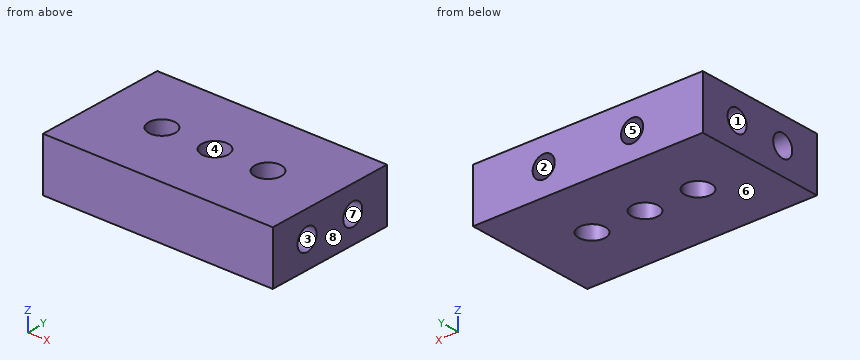
```python
from build123d import *

# Parameters (mm, degrees)
SKETCH_1_W                  = 26
SKETCH_1_H                  = 15
EXTRUDE_1_DEPTH             = 5
SKETCH_2_W                  = 26
SKETCH_2_H                  = 15
EXTRUDE_2_DEPTH             = 1
HOLE_WIZARD_M3_1_AT_2_COUNT = 2
HOLE_WIZARD_M3_1_AT_2_PITCH = 6
SKETCH_5_R                  = 1.5
CUT_EXTRUDE_1_DEPTH         = 7
HOLE_WIZARD_M3_2_D          = 2.5
HOLE_WIZARD_M3_2_DEPTH      = 7
HOLE_WIZARD_M3_2_TIP        = 0.751075774


with BuildPart() as part:
    # 草图1 → 凸台-拉伸1 (new body)
    with BuildSketch(Plane.XY):
        Rectangle(SKETCH_1_W, SKETCH_1_H)
    extrude(amount=EXTRUDE_1_DEPTH)

    # 草图2 → 凸台-拉伸2 (add)
    with BuildSketch(Plane.XY.offset(5)):
        Rectangle(SKETCH_2_W, SKETCH_2_H)
    extrude(amount=EXTRUDE_2_DEPTH)

    # 草图4 → M3 螺纹孔1 (revolve, cut)
    with BuildSketch(Plane(origin=(-13, -3, 3), x_dir=(0, 0, 1), z_dir=(0, 1, 0))):
        Polygon((0, 0), (0, 5.751075774), (1.25, 5), (1.25, 0), align=None)
    hole_wizard_m3_1 = revolve(axis=Axis((-19.35, -3, 3), (1, 0, 0)), mode=Mode.SUBTRACT)

    # M3 螺纹孔1 at 2: M3 螺纹孔1 ×2
    with Locations(*[(0, i * HOLE_WIZARD_M3_1_AT_2_PITCH, 0) for i in range(1, HOLE_WIZARD_M3_1_AT_2_COUNT)]):
        add(hole_wizard_m3_1, mode=Mode.SUBTRACT)

    # 镜向1: M3 螺纹孔1 across plane
    add(hole_wizard_m3_1.mirror(Plane(origin=(0, 0, 0), x_dir=(0, 0, 1), z_dir=(1, 0, 0))), mode=Mode.SUBTRACT)

    # 镜向1 copy 1 sketch → 镜向1 copy 1 (revolve, cut)
    with BuildSketch(Plane(origin=(13, 3, 3), x_dir=(0, 0, 1), z_dir=(0, 1, 0))):
        Polygon((0, 0), (0, -5.751075774), (1.25, -5), (1.25, 0), align=None)
    revolve(axis=Axis((19.35, 3, 3), (1, 0, 0)), mode=Mode.SUBTRACT)

    # 草图5 → 切除-拉伸1 (cut)
    with BuildSketch(Plane(origin=(0, 0, 0), x_dir=(-1, 0, 0), z_dir=(0, 0, -1))):
        with Locations((6, 0)):
            Circle(SKETCH_5_R)
        Circle(SKETCH_5_R)
        with Locations((-6, 0)):
            Circle(SKETCH_5_R)
    extrude(amount=-CUT_EXTRUDE_1_DEPTH, mode=Mode.SUBTRACT)

    # M3 螺纹孔2
    with Locations(Plane(origin=(5, 7.5, 3), x_dir=(0, 0, 1), z_dir=(0, 1, 0))):
        with Locations((0, 0), (0, -10)):
            Hole(HOLE_WIZARD_M3_2_D / 2, depth=HOLE_WIZARD_M3_2_DEPTH)
            with Locations((0, 0, -(HOLE_WIZARD_M3_2_DEPTH + HOLE_WIZARD_M3_2_TIP / 2))):  # 118° drill point
                Cone(0, HOLE_WIZARD_M3_2_D / 2, HOLE_WIZARD_M3_2_TIP, mode=Mode.SUBTRACT)


solid = part.part
```
Geometry check sheet. Reference: the model listing, model coordinates, mm. Face numbers are marked on the shaded views. A direction names the side the tool comes from. Give positions to 0.01 mm unless a question says otherwise; leave off trailing zeros. Write each loop counter-clockwise with the first axis right and the second up, starting at its lowest first coordinate (ties: lowest second). Pieces come first, ordered by that corner, then holes. Notation, with made-up numbers: (66, -40) -> (78, -40) arc R24 ccw to (78, -14) -> close; hole circle Ø3 at (11.25, -17.75). An arc over 180 degrees is marked (long way). Use one line per item in the form item = value.
Item 1: Access from +Z, -Z, +X, -X, +Y, -Y to the whole of each face (thin tool, end or side, straight path). Record for the marked faces 1, 2, 3 and 4.
Results list:
face_1 = -X
face_2 = +Y
face_3 = +X
face_4 = +Z, -Z
Item 2: Depth check by flat-ended pin: pin 1 Ø2 at (y, z) = (-3, 3) entering from -X; pin 2 Ø1 at (x, z) = (-4.5, 2.5) entering from +Y; pin 3 Ø2 at (y, z) = (-3, 3) entering from +X. Enter the tip coordinate at first touch or a pass-through.
Results list:
pin_1 = -7.85
pin_2 = 0.47
pin_3 = 7.85
Item 3: Scan lines: line 1 (Y direction, x = -9.5, z = 3); line 2 (X direction, y = 1.25, z = 3.25); line 3 (X direction, y = 5.75, z = 3). Record each from-to range of solid material in increasing order.
Results list:
line_1 = -7.5 to -4.25, -1.75 to 1.75, 4.25 to 7.5
line_2 = -13 to -6.83, -3.78 to -0.83, 0.83 to 3.78, 6.83 to 13
line_3 = -13 to -6.25, -3.75 to 3.75, 6.25 to 13
Item 4: Sectioned sample at B-B on x = 0. Enter the section's corners in (y, z), plus the area to 3 significant figures.
Results list:
outline = (-7.5, 0) -> (-1.5, 0) -> (-1.5, 6) -> (-7.5, 6) -> close; (1.5, 0) -> (7.5, 0) -> (7.5, 6) -> (1.5, 6) -> close
area = 72.0 mm2
Item 5: Sectioned sample at A-A on x = 6. Enter the section's corners in (y, z).
Results list:
outline = (-7.5, 0) -> (-1.5, 0) -> (-1.5, 6) -> (-7.5, 6) -> close; (1.5, 0) -> (7.5, 0) -> (7.5, 2.25) -> (1.5, 2.25) -> close; (1.5, 3.75) -> (7.5, 3.75) -> (7.5, 6) -> (1.5, 6) -> close
Item 6: Sectioned sample at D-D on y = 4. Count the separate pieces of the cut face and the enclosed holes in it, plus the area to 3 significant figures.
Results list:
separate_pieces = 1
enclosed_holes = 2
area = 131 mm2
Item 7: Sectioned sample at C-C on z = 0.75. Enter the section's corners in (x, y), plus the area to 3 significant figures.
Results list:
outline = (-13, -7.5) -> (13, -7.5) -> (13, 7.5) -> (-13, 7.5) -> close; hole circle Ø3 at (-6, 0); hole circle Ø3 at (0, 0); hole circle Ø3 at (6, 0)
area = 369 mm2
Item 8: Mould release check, pull along Z, two halves, no side actions. Record for the marked faces 5, 6, 7 and 8: released by +Z, released by -Z, zero draft, split by the parting line, or undercut.
Results list:
face_5 = undercut
face_6 = released by -Z
face_7 = undercut
face_8 = zero draft
